Input: dimensioned drawing with shaded views. Units: mm. Origin: part minimum x, y, z. Give positions to 0.01 mm unless a question says otherwise; leave off trailing zeros. Write each loop counter-clockwise with the first axis right and the second up, starting at its lowest first coordinate (ties: lowest second). Pieces come first, ordered by that corner, then holes.
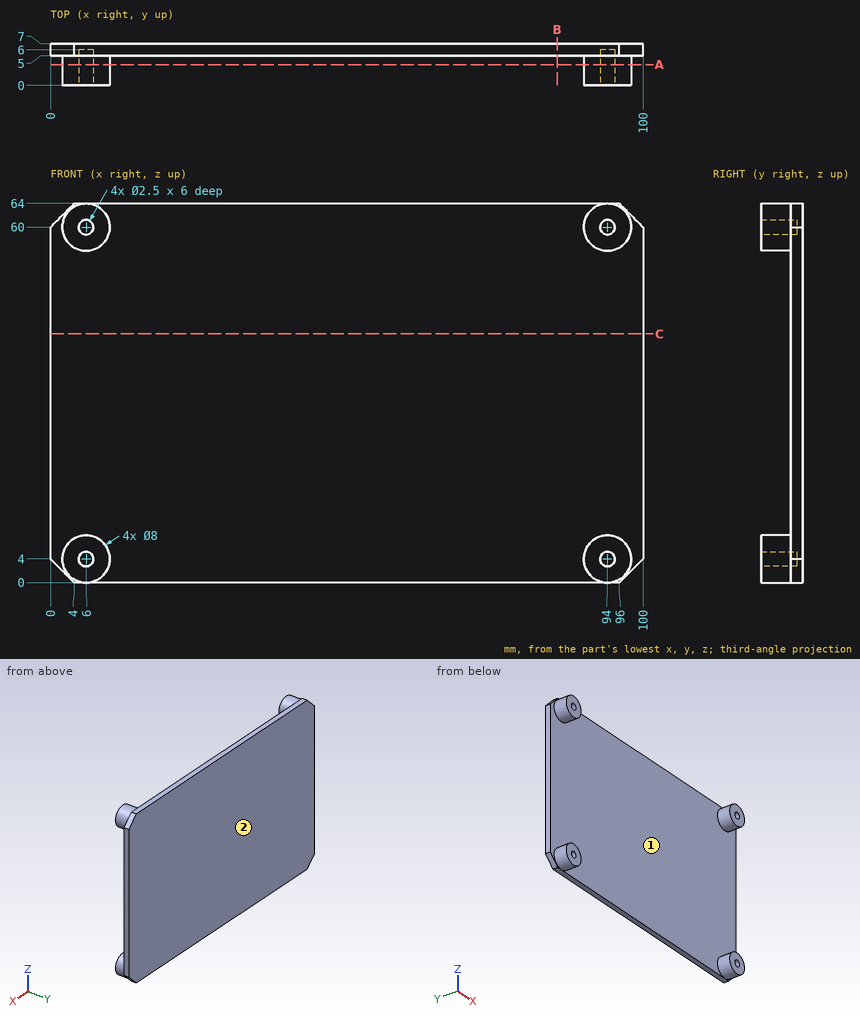
1. Line query: L1, parallel to X at y = 1.8, z = 4; L2, parallel to Z at x = 94, y = 4.1; L3, parallel to Y at x = 66.5, z = 18. Output: solid intervals per line, ascending.
2. Mould query, pull axis X, two halves, no side actions, for the marked faces 1 and 2. Classes: +X half, -X half, draft (parallel to the pull), parting line (faces both ways), or undercut.
3. Cut plane A-A, the plane y = 3.5. Return the cut outline in (x, z), then the cut area to 3 significant figures.
4. Cut plane C-C, the plane z = 42. Return the cut outline in (x, y), then the cut area to 3 significant figures.
5. Cut plane B-B, the plane x = 85.5. Return the cut outline in (y, z), then the cut area to 3 significant figures.
6. Contact query for flat-ended pins moving along their axis: P1, Ø2, axis at y = 2.5, z = 20.5, coming from the +X side; P2, Ø3, axis at x = 6, z = 4.5, coming from the -Y side; P3, Ø2, axis at x = 94, z = 4, coming from the -Y side; P4, Ø4, axis at x = 62, z = 40, coming from the -Y side. Output: stop coordinate, or through.
Response values:
1. L1: x = 2 to 4.75, 7.25 to 10, 90 to 92.75, 95.25 to 98
1. L2: z = 0 to 2.75, 5.25 to 8, 56 to 58.75, 61.25 to 64
1. L3: y = 5 to 7
2. face 1: undercut
2. face 2: draft
3. outline: circle Ø8 at (6, 4); circle Ø8 at (6, 60); circle Ø8 at (94, 4); circle Ø8 at (94, 60); hole circle Ø2.5 at (6, 4); hole circle Ø2.5 at (6, 60); hole circle Ø2.5 at (94, 4); hole circle Ø2.5 at (94, 60)
3. area: 181 mm2
4. outline: (0, 5) - (100, 5) - (100, 7) - (0, 7) - close
4. area: 200 mm2
5. outline: (5, 0) - (7, 0) - (7, 64) - (5, 64) - close
5. area: 128 mm2
6. P1: passes through
6. P2: stops at y = 0
6. P3: stops at y = 6
6. P4: stops at y = 5
